```python
from build123d import *

# Parameters (mm, degrees)
F1_DEPTH = 20
F2_SIZE  = 19.99999


# Not quite as in the source:
# - a fillet or chamfer is up to 0.001 mm smaller than in the source, because OpenCascade refuses the exact size


with BuildPart() as f1:
    # F0 (on Front) → F1 (new body)
    with BuildSketch(Plane.XZ):
        with BuildLine():
            Line((-129.9038105677, 75), (-43.3012701892, 25))
            ThreePointArc((-43.3012701892, 25), (-50, 0), (-43.3012701892, -25))
            Line((-43.3012701892, -25), (-129.9038105677, -75))
            ThreePointArc((-129.9038105677, -75), (-75, -129.9038105677), (0, -150))
            Line((0, -150), (0, -50))
            ThreePointArc((0, -50), (25, -43.3012701892), (43.3012701892, -25))
            Line((43.3012701892, -25), (129.9038105677, -75))
            ThreePointArc((129.9038105677, -75), (150, 0), (129.9038105677, 75))
            Line((129.9038105677, 75), (43.3012701892, 25))
            ThreePointArc((43.3012701892, 25), (25, 43.3012701892), (0, 50))
            Line((0, 50), (0, 150))
            ThreePointArc((0, 150), (-75, 129.9038105677), (-129.9038105677, 75))
        make_face()
        with BuildLine():
            ThreePointArc((-9.8107084352, -18), (-20.5, 0), (-9.8107084352, 18))
            Line((-9.8107084352, 18), (9.8107084352, 18))
            ThreePointArc((9.8107084352, 18), (20.5, 0), (9.8107084352, -18))
            Line((9.8107084352, -18), (-9.8107084352, -18))
        make_face(mode=Mode.SUBTRACT)
    extrude(amount=F1_DEPTH)

    # F2 (size 20 in the source; OpenCascade refuses exactly that, so slightly less here)
    f2_edges = [f1.edges().sort_by_distance(p)[0] for p in [
        (-86.60254, -20, 50),
        (0, -20, -100),
        (86.60254, -20, 50),
    ]]
    chamfer(f2_edges, length=F2_SIZE)


solid = f1.part
```
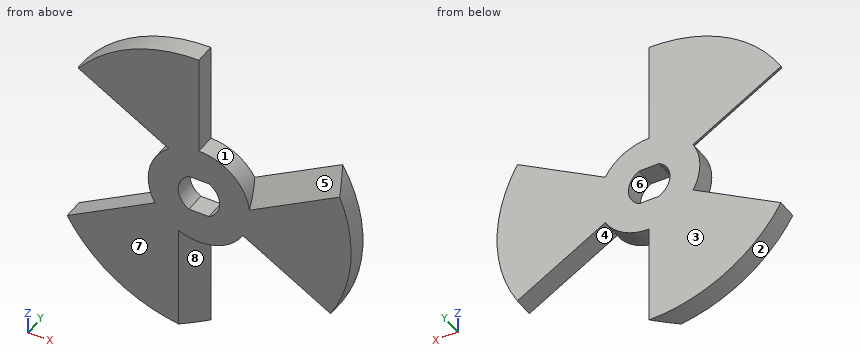
Build history of the part. All positions in model axes, mm. Face numbers are marked on the shaded views. A direction names the side the tool comes from. Give positions to 0.01 mm unless a question says otherwise; leave off trailing zeros. Loops run counter-clockwise (first coordinate to the right, second up) from the corner with the lowest first, then second, coordinate; pieces in that order, holes last.
Item 1: Slice it at B-B, the plane z = -5. List the corners of the cut face in (x, y), and give its area (3 significant figures).
Answers follow:
outline: (-49.75, -20) - (-19.88, -20) - (-19.88, 0) - (-49.75, 0) - close; (19.88, -20) - (149.92, -20) - (149.92, 0) - (19.88, 0) - close
area: 3,200 mm2
Item 2: Slice it at C-C, the plane y = -10.75. List the corners of the cut face in (x, z).
Answers follow:
outline: (-129.9, -75) arc R150 ccw to (-10.75, -149.61) - (-10.75, -48.83) arc R50 ccw to (43.3, -25) - (129.9, -75) arc R150 ccw to (134.94, 65.5) - (47.66, 15.11) arc R50 ccw to (0, 50) - (0, 150) arc R150 ccw to (-124.19, 84.12) - (-36.91, 33.73) arc R50 ccw to (-43.3, -25) - close; hole (-9.81, -18) - (9.81, -18) arc R20.5 ccw to (9.81, 18) - (-9.81, 18) arc R20.5 ccw to start
Item 3: Pull direction X, two halves, no side cores. Call the marked faces 1, 2 and 3: released by +X, released by -X, zero draft, split by the parting line, or undercut.
Answers follow:
face 1: undercut
face 2: released by -X
face 3: zero draft
Item 4: Slice it at D-D, the plane z = 79. List the corners of the cut face in (x, y), and give its area (3 significant figures).
Answers follow:
outline: (-127.51, -4.66) - (-96.83, -20) - (0, -20) - (0, 0) - (-127.51, 0) - close
area: 2,310 mm2
Item 5: Which spindle directions (+Z, -Z, +X, -X, +Y, -Y) get a long thin tool onto all of the face, cutting with end or side? Do the marked faces 4, 5, 6, 7 and 8. Say none if no direction does.
Answers follow:
face 4: -Z, +Y, -Y
face 5: +Z, -Y
face 6: +Y, -Y
face 7: +Z, -Z, +X, -X, -Y
face 8: -Z, -Y
Item 6: Flat gauge pins, fed straight in: pin 1 (4 mm diameter, centred on x = -76, z = -52.5, fed in from +Y); pin 2 (5 mm diameter, centred on x = -39.5, y = -15.5, fed in from -Z); pin 3 (6 mm diameter, centred on y = -14, z = 79, fed in from +X); pin 4 (12 mm diameter, centred on x = 43.5, y = -3.5, fed in from -Z). Where does each tip first touch, or does it go through?
Answers follow:
pin 1: stops at y = 0
pin 2: stops at z = -145.37
pin 3: stops at x = 0
pin 4: stops at z = -33.07
Item 7: Drill centre lines: line 1 (X direction, y = -16.5, z = 12.5); line 2 (X direction, y = -6.75, z = 1); line 3 (X direction, y = -16.75, z = 4.5). Where is each one in solid material? Low to high.
Answers follow:
line 1: x = -48.41 to -16.25, 16.25 to 48.41, 54.65 to 149.48
line 2: x = -49.99 to -20.48, 20.48 to 150
line 3: x = -49.8 to -20, 20 to 149.93
